```python
from build123d import *

# Parameters (mm, degrees)
BOSS_EXTRUDE1_DEPTH = 3


with BuildPart() as part:
    # Sketch1 → Boss-Extrude1 (new body)
    with BuildSketch(Plane(origin=(0, 0, 0), x_dir=(1, 0, 0), z_dir=(0, 1, 0))):
        with BuildLine():
            Line((0, 6), (0, 12.885607037))
            ThreePointArc((0, 12.885607037), (-0.594451952, 14.983759198), (-2.201121246, 16.458286036))
            Line((-2.201121246, 16.458286036), (-4.154505591, 17.441834123))
            ThreePointArc((-4.154505591, 17.441834123), (-9.586112213, 19.258544509), (-15.309892207, 19.461349126))
            Line((-15.309892207, 19.461349126), (-19.293684392, 19.028366911))
            ThreePointArc((-19.293684392, 19.028366911), (-20.375358342, 18.473602904), (-20.81, 17.338319562))
            Line((-20.81, 17.338319562), (-20.81, 16.238803173))
            Line((-20.81, 16.238803173), (-11.03, 14.16))
            ThreePointArc((-11.03, 14.16), (-9.874646135, 12.380911063), (-11.653735072, 11.225557198))
            Line((-11.653735072, 11.225557198), (-20.81, 13.171781389))
            Line((-20.81, 13.171781389), (-20.81, 4.766752866))
            ThreePointArc((-20.81, 4.766752866), (-20.567080075, 1.086466776), (-19.842535307, -2.529961112))
            ThreePointArc((-19.842535307, -2.529961112), (-19.024517018, -3.911631932), (-17.611135307, -4.673550768))
            ThreePointArc((-17.611135307, -4.673550768), (-14.527545315, -5.195342958), (-11.405, -5.37))
            Line((-11.405, -5.37), (-2, -5.37))
            ThreePointArc((-2, -5.37), (-0.585786438, -4.784213562), (0, -3.37))
            Line((0, -3.37), (0, 0))
            Line((0, 0), (-10.03, 0))
            ThreePointArc((-10.03, 0), (-10.737106781, 0.292893219), (-11.03, 1))
            Line((-11.03, 1), (-11.03, 5))
            ThreePointArc((-11.03, 5), (-10.737106781, 5.707106781), (-10.03, 6))
            Line((-10.03, 6), (0, 6))
        make_face()
    extrude(amount=BOSS_EXTRUDE1_DEPTH)


solid = part.part
```
Verification items for the finished model (mm, model axes). A direction names the side the tool comes from. Coordinates: 2 decimals unless noted, no trailing zeros. Loops run counter-clockwise (first coordinate to the right, second up) from the corner with the lowest first, then second, coordinate; pieces in that order, holes last. Notation, with made-up numbers: (79, 14.5) -> (115, 14.5) arc R20 cw to (115, 48.5) -> close; hole circle Ø6 at (-31, -3.75). An arc over 180 degrees is marked (long way). Answer in a Markdown table with one row per item.
1) Access from +Z, -Z, +X, -X, +Y, -Y to the whole of each face (thin tool, end or side, straight path). Record for faces 4 (the face through (-15.988, 1.479, -15.214)), 5 (the face through (-11.03, 1, -3)), 6 (the face through (0, 1, -9)).
The answers:
| item | result |
|---|---|
| face 4 | -X, +Y, -Y |
| face 5 | +X, +Y, -Y |
| face 6 | +Z, -Z, +X, +Y, -Y |
2) Section check B-B (y = 1.05). Record the cut outline in (x, z) (1 decimal), and give its area (3 significant figures).
The answers:
| item | result |
|---|---|
| outline | (-20.8, -17.3) arc R1.7 ccw to (-19.3, -19) -> (-15.3, -19.5) arc R20 ccw to (-4.2, -17.4) -> (-2.2, -16.5) arc R4 ccw to (0, -12.9) -> (0, -6) -> (-10, -6) arc R1 cw to (-11, -5) -> (-11, -1) arc R1 cw to (-10, 0) -> (0, 0) -> (0, 3.4) arc R2 ccw to (-2, 5.4) -> (-11.4, 5.4) arc R28 ccw to (-17.6, 4.7) arc R3 ccw to (-19.8, 2.5) arc R28 ccw to (-20.8, -4.8) -> (-20.8, -13.2) -> (-11.7, -11.2) arc R1.5 cw to (-11, -14.2) -> (-20.8, -16.2) -> close |
| area | 387 mm2 |
3) Draft check along Z on faces 1 (the face through (-19.041, 1.479, 3.896)), 2 (the face through (-11, 0, -7)), 3 (the face through (-10.729, 1.479, -0.285)). Enter one of: released by +Z, released by -Z, zero draft, split by the parting line, or undercut.
The answers:
| item | result |
|---|---|
| face 1 | released by +Z |
| face 2 | zero draft |
| face 3 | undercut |
4) Depth check by flat-ended pin: P1, Ø1.5, axis at x = -7, y = 1, coming from the -Z side; P2, Ø0.9, axis at y = 1.5, z = -3.5, coming from the +X side. Enter the tip coordinate at first touch or a pass-through.
The answers:
| item | result |
|---|---|
| P1 | stops at z = -18.84 |
| P2 | stops at x = -11.03 |
5) Scan lines: line 1 along Z through (x, y) = (-8.5, 0.4); line 2 along Z through (x, y) = (-15, 1.1); line 3 along X through (y, z) = (1.1, -4.5). Record each from-to range of solid material in increasing order. Write a range as from..to.
The answers:
| item | result |
|---|---|
| line 1 | z = -19.03..-6, 0..5.37 |
| line 2 | z = -19.49..-15, -11.94..5.14 |
| line 3 | x = -20.81..-11.03 |
6) Section check D-D (z = 2). Record the cut outline in (x, y), and give its area (3 significant figures).
The answers:
| item | result |
|---|---|
| outline | (-19.98, 0) -> (0, 0) -> (0, 3) -> (-19.98, 3) -> close |
| area | 59.9 mm2 |
7) Section check A-A (x = -12.5). Record the cut outline in (y, z).
The answers:
| item | result |
|---|---|
| outline | (0, -19.57) -> (3, -19.57) -> (3, -14.47) -> (0, -14.47) -> close; (0, -11.41) -> (3, -11.41) -> (3, 5.35) -> (0, 5.35) -> close |
8) Section check C-C (x = -14.75). Record the cut outline in (y, z), and give its area (4 significant figures).
The answers:
| item | result |
|---|---|
| outline | (0, -19.51) -> (3, -19.51) -> (3, -14.95) -> (0, -14.95) -> close; (0, -11.88) -> (3, -11.88) -> (3, 5.17) -> (0, 5.17) -> close |
| area | 64.85 mm2 |
